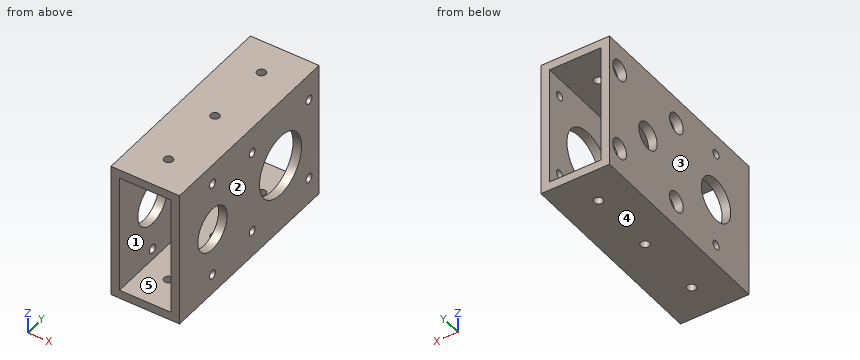
Autodesk Inventor part; units mm, degrees
ref_plane "YZ Plane" through (0, 0, 0) normal (1, 0, 0) x (0, 1, 0)
ref_plane "XZ Plane" through (0, 0, 0) normal (0, 1, 0) x (-1, 0, 0)
ref_plane "XY Plane" through (0, 0, 0) normal (0, 0, 1) x (1, 0, 0)
sketch "Sketch1" plane through (0, 0, 0) normal (0, 1, 0) x (-1, 0, 0)
  line L0 (-12.7, 25.4) -> (12.7, 25.4)
  line L1 (12.7, 25.4) -> (12.7, -25.4)
  line L2 (12.7, -25.4) -> (-12.7, -25.4)
  line L3 (-12.7, -25.4) -> (-12.7, 25.4)
  line L4 (-12.7, 25.4) -> (12.7, -25.4) construction
  line L5 (12.7, 25.4) -> (-12.7, -25.4) construction
  point P0 (0, 0)
  dimension "d0" = 50.8
  dimension "d1" = 25.4
extrude "Extrusion1" add sketch "Sketch1" along normal blind 76.2
shell "Shell1" thickness 3.175 removed faces 2 at (-4.2333, 0, 8.4667) at (-4.2333, 76.2, 8.4667)
sketch "Sketch2" plane through (-12.7, 0, -25.4) normal (-1, 0, 0) x (0, 0, 1)
  line L0 (9.9, 39.7) -> (40.9, 39.7)
  line L1 (40.9, 39.7) -> (40.9, 70.7)
  line L2 (40.9, 70.7) -> (9.9, 70.7)
  line L3 (9.9, 70.7) -> (9.9, 39.7)
  line L4 (9.9, 39.7) -> (40.9, 70.7) construction
  line L5 (40.9, 39.7) -> (9.9, 70.7) construction
  line L6 (0, 76.2) -> (50.8, 76.2)
  point P0 (25.4, 0)
  point P1 (25.4, 55.2)
  point P2 (25.4, 55.2)
  point P3 (25.4, 76.2)
  dimension "d5" = 31
  dimension "d6" = 31
  dimension "d7" = 21
hole "Hole1" at (-12.7, 70.7, -15.5) at (-12.7, 70.7, 15.5) at (-12.7, 39.7, 15.5) at (-12.7, 39.7, -15.5) direction (1, 0, 0) diameter 3.2 end through all counterbore diameter 7.5 counterbore depth 5
hole "Hole2" at (-12.7, 55.2, 0) direction (1, 0, 0) diameter 10 end through all
sketch "Sketch3" plane through (12.7, 0, 25.4) normal (1, 0, 0) x (0, 0, -1)
  circle A0 centre (25.4, 55.2) radius 5
  circle A1 centre (25.4, 55.2) radius 11.5
  point P0 (25.4, 0)
  dimension "d22" = 23
extrude "Extrusion2" cut sketch "Sketch3" against normal up to surface (22.225 mm away) contours A0 | A1
sketch "Sketch4" plane through (12.7, 0, 25.4) normal (1, 0, 0) x (0, 0, -1)
  circle A0 centre (25.4, 18) radius 8
  line L0 (50.8, 0) -> (0, 0)
  point P0 (25.4, 0)
  point P1 (25.4, 0)
  dimension "d25" = 16
  dimension "d26" = 18
extrude "Extrusion3" cut sketch "Sketch4" against normal through all
sketch "Sketch6" plane through (12.7, 0, -25.4) normal (0, 0, -1) x (-1, 0, 0)
  line L0 (12.7, 12.7) -> (12.7, 63.5)
  line L1 (25.4, 0) -> (0, 0)
  line L2 (0, 76.2) -> (25.4, 76.2)
  line L3 (25.4, 0) -> (25.4, 76.2)
  point P0 (12.7, 0)
  point P1 (12.7, 38.1)
  point P2 (12.7, 0)
  point P3 (25.4, 38.1)
  dimension "d55" = 50.8
hole "Hole4" at (0, 38.1, -25.4) at (0, 63.5, -25.4) at (0, 12.7, -25.4) direction (0, 0, 1) diameter 3.242 end through all
sketch "Sketch7" plane through (12.7, 0, 25.4) normal (1, 0, 0) x (0, 0, -1)
  circle A0 centre (25.4, 18) radius 8
  line L0 (7.4, 18) -> (43.4, 18)
  point P0 (25.4, 0)
  dimension "d47" = 36
hole "Hole5" at (12.7, 18, -18) at (12.7, 18, 18) direction (-1, 0, 0) diameter 3.242 end through all
equation "\"d6\" = d5"
properties part number "Transmission_Case"
Geometry: final body of the model. Coordinates: model frame, mm. Face numbers are marked on the shaded views. A direction names the side the tool comes from. Give positions to 0.01 mm unless a question says otherwise; leave off trailing zeros. Loops run counter-clockwise (first coordinate to the right, second up) from the corner with the lowest first, then second, coordinate; pieces in that order, holes last. Notation, with made-up numbers: (37.5, 28) -> (48.5, 28) arc R23 cw to (48.5, 61) -> close; hole circle Ø6 at (20.5, -0.75). An arc over 180 degrees is marked (long way). Put each result on its own line as item: value.
1. Cut plane C-C (z = -15.5). Return the cut outline in (x, y) (3 decimals).
Taken from the geometry:
outline: (-12.7, 0) -> (-9.525, 0) -> (-9.525, 35.95) -> (-12.7, 35.95) -> close; (-12.7, 43.45) -> (-9.525, 43.45) -> (-9.525, 66.95) -> (-12.7, 66.95) -> close; (-12.7, 74.45) -> (-9.525, 74.45) -> (-9.525, 76.2) -> (-12.7, 76.2) -> close; (9.525, 0) -> (12.7, 0) -> (12.7, 38.1) -> (9.525, 38.1) -> close; (9.525, 41.3) -> (12.7, 41.3) -> (12.7, 69.1) -> (9.525, 69.1) -> close; (9.525, 72.3) -> (12.7, 72.3) -> (12.7, 76.2) -> (9.525, 76.2) -> close
2. Ray query, line 1 along Y through (x, z) = (0, -23.6); line 2 along Y through (x, z) = (-10.65, -15.5); line 3 along Y through (x, z) = (10.35, 15.5). Return the intervals inside material, ascending. Write a range as [from, to].
Taken from the geometry:
line 1: y = [0, 11.08], [14.32, 36.48], [39.72, 61.88], [65.12, 76.2]
line 2: y = [0, 35.95], [43.45, 66.95], [74.45, 76.2]
line 3: y = [0, 38.1], [41.3, 69.1], [72.3, 76.2]
3. Cut plane A-A (y = 18). Count the separate pieces of the cut face and the enclosed holes in it, plus the area to 3 significant figures.
Taken from the geometry:
separate pieces: 6
enclosed holes: 0
area: 301 mm2
4. Cut plane B-B (x = -8.75). Return the cut outline in (y, z) (3 decimals), plus the area to 3 significant figures.
Taken from the geometry:
outline: (0, -25.4) -> (76.2, -25.4) -> (76.2, -22.225) -> (0, -22.225) -> close; (0, 22.225) -> (76.2, 22.225) -> (76.2, 25.4) -> (0, 25.4) -> close
area: 484 mm2
5. Pin query (flat end, axial travel): P1, Ø6, axis at y = 70.7, z = 15.5, coming from the -X side (3 decimals); P2, Ø3, axis at x = -7, z = 2, coming from the -Y side. Return the tip coordinate at first contact, or that it passes through.
Taken from the geometry:
P1: stops at x = 9.525
P2: passes through
6. Pull-direction query (X, two-part tool) for the marked faces 3, 4 and 5; classes: released by +X, released by -X, zero draft, split by the parting line, or undercut.
Taken from the geometry:
face 3: released by -X
face 4: zero draft
face 5: undercut
7. Set-up query: the marked faces 1 and 2. Return all of +Z, -Z, +X, -X, +Y, -Y with unobstructed straight access to the full face (end or side cutting, diameter ignored); none if empty.
Taken from the geometry:
face 1: +Y, -Y
face 2: +Z, -Z, +X, +Y, -Y
